```python
from build123d import *

# Parameters (mm, degrees)
SKETCH1_W                                            = 300
SKETCH1_H                                            = 50
SKETCH1_R                                            = 4
MAIN_DEPTH                                           = 10
SKETCH4_R                                            = 2.5
MOUNT_DEPTH                                          = 11
SKETCH2_R                                            = 11
SKETCH2_R_2                                          = 1.5
STEPPER_MOUNT_DEPTH                                  = 11
CSK_FOR_M6_SOCKET_COUNTERSUNK_HEAD_SCREW_D           = 6.6
CSK_FOR_M6_SOCKET_COUNTERSUNK_HEAD_SCREW_DEPTH       = 15
CSK_FOR_M6_SOCKET_COUNTERSUNK_HEAD_SCREW_CSINK_D     = 13.71
CSK_FOR_M6_SOCKET_COUNTERSUNK_HEAD_SCREW_CSINK_ANGLE = 90
CSK_FOR_M6_SOCKET_COUNTERSUNK_HEAD_SCREW_TIP         = 1.982840043
CSK_FOR_M3_SOCKET_COUNTERSUNK_HEAD_SCREW_D           = 3.4
CSK_FOR_M3_SOCKET_COUNTERSUNK_HEAD_SCREW_DEPTH       = 15
CSK_FOR_M3_SOCKET_COUNTERSUNK_HEAD_SCREW_CSINK_D     = 6.94
CSK_FOR_M3_SOCKET_COUNTERSUNK_HEAD_SCREW_CSINK_ANGLE = 90
CSK_FOR_M3_SOCKET_COUNTERSUNK_HEAD_SCREW_TIP         = 1.021463052


with BuildPart() as part:
    # Sketch1 → main (new body)
    with BuildSketch(Plane(origin=(0, 0, 0), x_dir=(1, 0, 0), z_dir=(0, 1, 0))):
        with Locations((0, -5)):
            Rectangle(SKETCH1_W, SKETCH1_H)
        with Locations((-100, 0)):
            Circle(SKETCH1_R, mode=Mode.SUBTRACT)
        with Locations((100, 0)):
            Circle(SKETCH1_R, mode=Mode.SUBTRACT)
    extrude(amount=MAIN_DEPTH)

    # Sketch4 → mount (cut, through all)
    with BuildSketch(Plane(origin=(0, 10, 0), x_dir=(1, 0, 0), z_dir=(0, 1, 0))):
        with Locations((-140, 5)):
            Circle(SKETCH4_R)
        with Locations((-140, -15)):
            Circle(SKETCH4_R)
        with Locations((140, -15)):
            Circle(SKETCH4_R)
        with Locations((140, 5)):
            Circle(SKETCH4_R)
    extrude(amount=-MOUNT_DEPTH, mode=Mode.SUBTRACT)

    # Sketch2 → stepper_mount (cut, through all)
    with BuildSketch(Plane(origin=(0, 10, 0), x_dir=(1, 0, 0), z_dir=(0, 1, 0))):
        with Locations((0, -1)):
            Circle(SKETCH2_R)
        with Locations((15.5, -16.5)):
            Circle(SKETCH2_R_2)
        with Locations((-15.5, -16.5)):
            Circle(SKETCH2_R_2)
        with Locations((-15.5, 14.5)):
            Circle(SKETCH2_R_2)
        with Locations((15.5, 14.5)):
            Circle(SKETCH2_R_2)
    extrude(amount=-STEPPER_MOUNT_DEPTH, mode=Mode.SUBTRACT)

    # CSK for M6 socket countersunk head screw1
    with Locations(Plane(origin=(0, 10, 0), x_dir=(1, 0, 0), z_dir=(0, 1, 0))):
        with Locations((140, -15), (140, 5), (-140, -15), (-140, 5)):
            CounterSinkHole(CSK_FOR_M6_SOCKET_COUNTERSUNK_HEAD_SCREW_D / 2, CSK_FOR_M6_SOCKET_COUNTERSUNK_HEAD_SCREW_CSINK_D / 2, depth=CSK_FOR_M6_SOCKET_COUNTERSUNK_HEAD_SCREW_DEPTH, counter_sink_angle=CSK_FOR_M6_SOCKET_COUNTERSUNK_HEAD_SCREW_CSINK_ANGLE)
            with Locations((0, 0, -(CSK_FOR_M6_SOCKET_COUNTERSUNK_HEAD_SCREW_DEPTH + CSK_FOR_M6_SOCKET_COUNTERSUNK_HEAD_SCREW_TIP / 2))):  # 118° drill point
                Cone(0, CSK_FOR_M6_SOCKET_COUNTERSUNK_HEAD_SCREW_D / 2, CSK_FOR_M6_SOCKET_COUNTERSUNK_HEAD_SCREW_TIP, mode=Mode.SUBTRACT)

    # CSK for M3 socket countersunk head screw1
    with Locations(Plane(origin=(0, 0, 0), x_dir=(-1, 0, 0), z_dir=(0, -1, 0))):
        with Locations((15.5, -16.5), (-15.5, -16.5), (-15.5, 14.5), (15.5, 14.5)):
            CounterSinkHole(CSK_FOR_M3_SOCKET_COUNTERSUNK_HEAD_SCREW_D / 2, CSK_FOR_M3_SOCKET_COUNTERSUNK_HEAD_SCREW_CSINK_D / 2, depth=CSK_FOR_M3_SOCKET_COUNTERSUNK_HEAD_SCREW_DEPTH, counter_sink_angle=CSK_FOR_M3_SOCKET_COUNTERSUNK_HEAD_SCREW_CSINK_ANGLE)
            with Locations((0, 0, -(CSK_FOR_M3_SOCKET_COUNTERSUNK_HEAD_SCREW_DEPTH + CSK_FOR_M3_SOCKET_COUNTERSUNK_HEAD_SCREW_TIP / 2))):  # 118° drill point
                Cone(0, CSK_FOR_M3_SOCKET_COUNTERSUNK_HEAD_SCREW_D / 2, CSK_FOR_M3_SOCKET_COUNTERSUNK_HEAD_SCREW_TIP, mode=Mode.SUBTRACT)


solid = part.part
```
Could you check a few things on this model? Use its own coordinates, in mm. Coordinates: 2 decimals unless noted, no trailing zeros. Order: outer loops, then holes, each group sorted by start corner. A loop starts at its lowest first (then second) coordinate and runs counter-clockwise, first axis right, second up. Notation, with made-up numbers: M -19,3 L -14,3 A25 ccw -14,29 Z; hole C 72.25,0 d1. An arc over 180 degrees is marked long. Use a Markdown table: item, result. Add a question column.
Q1. We'd pull the mould along X, two halves only. Please class faces 1 (the flat face through (-2, 0, 16)), 2 (the conical face through (-143.312, 6.618, -6.043)): pulls with the +X half, pulls with the -X half, needs draft (parallel to the pull), parting line crosses it, or undercut.
Q2. I'm going to push flat-ended pins straight in: pin 1 (4.5 mm diameter, centred on x = 15.5, z = 16.5, fed in from -Y); pin 2 (7.5 mm diameter, centred on x = 140, z = -5, fed in from +Y) (3 decimals); pin 3 (8.5 mm diameter, centred on x = 140, z = 15, fed in from +Y) (3 decimals). Where does each tip first touch, or does it pass through?
Q3. I want a section at A-A on x = -140. List the corners of the cut face in (y, z) for me (3 decimals).
Q4. If I drill on L1, parallel to Z at x = -140, y = 1.75; L2, parallel to X at y = 4.25, z = -14.5; L3, parallel to X at y = 4.25, z = 15, over which ranges is the centre line in solid material (lowest first)?
Q5. I want a section at B-B on x = -100. List the corners of the cut face in (y, z) for me, then the cut area to 3 significant figures.
Q6. I want a section at C-C on x = 0. List the corners of the cut face in (y, z) for me.
Checked values:
| question | item | result |
|---|---|---|
| 1 | face 1 | needs draft |
| 1 | face 2 | undercut |
| 2 | pin 1 | y = 1.22 |
| 2 | pin 2 | y = 6.895 |
| 2 | pin 3 | y = 7.395 |
| 3 | outline | M 0,-20 L 10,-20 L 10,-11.855 L 6.445,-8.3 L 0,-8.3 Z; M 0,-1.7 L 6.445,-1.7 L 10,1.855 L 10,8.145 L 6.445,11.7 L 0,11.7 Z; M 0,18.3 L 6.445,18.3 L 10,21.855 L 10,30 L 0,30 Z |
| 4 | L1 | -20 to -8.3, -1.7 to 11.7, 18.3 to 30 |
| 4 | L2 | -150 to -17.2, -13.8 to 13.8, 17.2 to 150 |
| 4 | L3 | -150 to -143.3, -136.7 to -16.3, -14.7 to 14.7, 16.3 to 136.7, 143.3 to 150 |
| 5 | outline | M 0,-20 L 10,-20 L 10,-4 L 0,-4 Z; M 0,4 L 10,4 L 10,30 L 0,30 Z |
| 5 | area | 420 mm² |
| 6 | outline | M 0,-20 L 10,-20 L 10,-10 L 0,-10 Z; M 0,12 L 10,12 L 10,30 L 0,30 Z |
